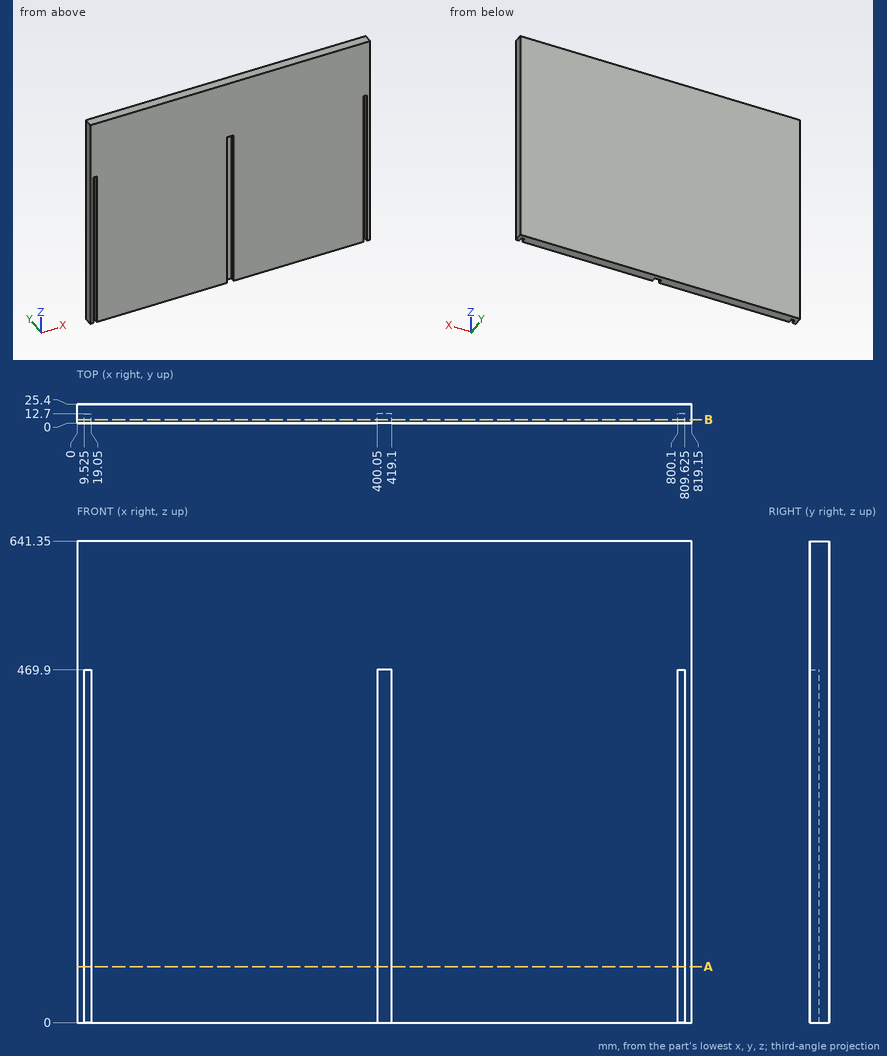
The drawing under review shows one solid part. Ordinate dimensions are in mm from its lowest x, y, z. Round coordinates to 2 decimals unless told otherwise and drop trailing zeros. Loops run counter-clockwise (first coordinate to the right, second up) from the corner with the lowest first, then second, coordinate; pieces in that order, holes last. Notation, with made-up numbers: (-33, 39.25) - (-29, 39.25) arc R31 ccw to (-29, 66.25) - close; hole circle Ø9 at (48.5, -14). An arc over 180 degrees is marked (long way). Put each result on its own line as item: value. Start each with the question number.
1. Consider section B-B on y = 4.75. State the section outline as (x, z) points (3 decimals), plus the area to 3 significant figures.
2. Consider section A-A on z = 74.5. State the section outline as (x, y) points (3 decimals).
3. For probe 1 along X at (y, z) = (10, 34.5) (3 decimals), list the stretches that pass through material, from the lowest coordinate up. Write a range as [from, to].
4. Insertion check: P1, Ø10, axis at y = 6, z = 252.5, coming from the -X side; P2, Ø3, axis at x = 806, z = 236, coming from the -Y side; P3, Ø6.5, axis at x = 406.5, y = 7.5, coming from the -Z side. Each pin has a flat end and moves straight along its axis. Give the tip position at first contact, or say it passes through.
Result sheet:
1. outline: (0, 0) - (9.525, 0) - (9.525, 469.9) - (19.05, 469.9) - (19.05, 0) - (400.05, 0) - (400.05, 469.9) - (419.1, 469.9) - (419.1, 0) - (800.1, 0) - (800.1, 469.9) - (809.625, 469.9) - (809.625, 0) - (819.15, 0) - (819.15, 641.35) - (0, 641.35) - close
1. area: 507,000 mm^2
2. outline: (0, 0) - (9.525, 0) - (9.525, 12.7) - (19.05, 12.7) - (19.05, 0) - (400.05, 0) - (400.05, 12.7) - (419.1, 12.7) - (419.1, 0) - (800.1, 0) - (800.1, 12.7) - (809.625, 12.7) - (809.625, 0) - (819.15, 0) - (819.15, 25.4) - (0, 25.4) - close
3. probe 1: [0, 9.525], [19.05, 400.05], [419.1, 800.1], [809.625, 819.15]
4. P1: x = 0
4. P2: y = 12.7
4. P3: z = 469.9
